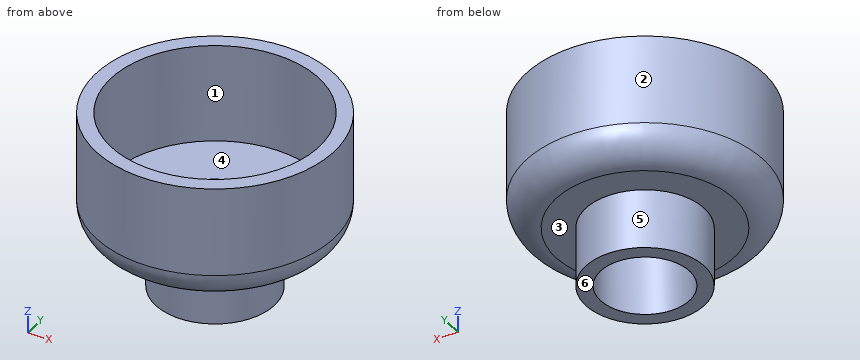
Autodesk Inventor part; units mm, degrees
ref_plane "YZ Plane" through (0, 0, 0) normal (1, 0, 0) x (0, 1, 0)
ref_plane "XZ Plane" through (0, 0, 0) normal (0, 1, 0) x (-1, 0, 0)
ref_plane "XY Plane" through (0, 0, 0) normal (0, 0, 1) x (1, 0, 0)
sketch "Sketch1" plane through (0, 0, 0) normal (0, 0, 1) x (1, 0, 0)
  circle A0 centre (0, 0) radius 40
  circle A1 centre (0, 0) radius 15
  dimension "d0" = 80
  dimension "d1" = 30
extrude "Extrusion1" add sketch "Sketch1" along normal blind 40
sketch "Sketch2" plane through (0, 0, 0) normal (0, 0, -1) x (-1, 0, 0)
  circle A0 centre (0, 0) radius 20
  dimension "d4" = 40
extrude "Extrusion2" add sketch "Sketch2" along normal blind 20
extrude "Extrusion3" cut sketch "Sketch1" against normal blind 20 contours A1
fillet "Fillet1" radius 10 1 edges at (-40, 0, 0)
sketch "Sketch3" plane through (0, 0, 40) normal (0, 0, 1) x (1, 0, 0)
  circle A0 centre (0, 0) radius 35
  dimension "d10" = 70
extrude "Extrusion4" cut sketch "Sketch3" against normal blind 33
properties part number "output"
Input: part model. Units: mm. Frame: model coordinates. Face numbers are marked on the shaded views. A direction names the side the tool comes from. Round coordinates to 2 decimals unless told otherwise and drop trailing zeros. Loops run counter-clockwise (first coordinate to the right, second up) from the corner with the lowest first, then second, coordinate; pieces in that order, holes last. Notation, with made-up numbers: (-26.5, 6) - (-12.5, 6) arc R27 cw to (-12.5, 26) - close; hole circle Ø9 at (17.25, 48.5). An arc over 180 degrees is marked (long way). One line per item, written item: value. Start each with the question number.
(1) Section D-D, the plane z = 32. Return loops of the section in (x, y), plus the area to 3 significant figures.
(2) Contact query for flat-ended pins moving along their axis: P1, Ø3, axis at x = -27, y = -7.5, coming from the -Z side; P2, Ø1, axis at y = -14.5, z = 2, coming from the +X side; P3, Ø2, axis at y = 17.5, z = 29, coming from the -X side. Output: stop coordinate, or through.
(3) Ray query, line 1 (Y direction, x = 0, z = 25.5); line 2 (Y direction, x = 0, z = -11); line 3 (Z direction, x = 15.5, y = -21). Return the intervals inside material, ascending. Write a range as [from, to].
(4) Draft query along X for the marked faces 4, 5 and 6. Return one class per face: +X half, -X half, draft (parallel to the pull), parting line (faces both ways), or undercut.
(5) Section C-C, the plane z = 4. Return loops of the section in (x, y).
(6) Section A-A, the plane y = 0. Return loops of the section in (x, z), plus the area to 3 significant figures.
(7) Access query for the marked faces 1, 2 and 3. Directions: +Z, -Z, +X, -X, +Y, -Y. A direction counts if a zero-diameter tool reaches every point of the face in a straight line with its end or side. Return the directions, or none.
Results below:
1. outline: circle Ø80 at (0, 0); hole circle Ø70 at (0, 0)
1. area: 1,180 mm^2
2. P1: z = 0
2. P2: x = 33.66
2. P3: x = -36.44
3. line 1: [-40, -35], [35, 40]
3. line 2: [-20, -15], [15, 20]
3. line 3: [0, 7]
4. face 4: undercut
4. face 5: parting line
4. face 6: draft
5. outline: circle Ø76 at (0, 0); hole circle Ø30 at (0, 0)
6. outline: (-40, 10) arc R10 ccw to (-30, 0) - (-20, 0) - (-20, -20) - (-15, -20) - (-15, 7) - (-35, 7) - (-35, 40) - (-40, 40) - close; (15, -20) - (20, -20) - (20, 0) - (30, 0) arc R10 ccw to (40, 10) - (40, 40) - (35, 40) - (35, 7) - (15, 7) - close
6. area: 837 mm^2
7. face 1: +Z
7. face 2: +Z, -Z
7. face 3: -Z
